For this review, take the finished solid that the model builds, in its own axes (mm). A direction names the side the tool comes from. Give positions to 0.01 mm unless a question says otherwise; leave off trailing zeros. Order: outer loops, then holes, each group sorted by start corner. A loop starts at its lowest first (then second) coordinate and runs counter-clockwise, first axis right, second up. Notation, with made-up numbers: M 57.5,-14 L 69.5,-14 A11 ccw 69.5,-8 Z; hole C -2,27.25 d3. An arc over 180 degrees is marked long. Use CSV: the item, a comma, the result in double quotes. Start each with the question number.
(1) Consider section B-B (x = 200). Give the number of separate pieces and of enclosed holes in the cut face, and give its area (3 significant figures).
(2) Consider section A-A (z = 32). Write out the cut boundary in (x, y), and give its area (3 significant figures).
(3) Consider section C-C (y = -329.5). Write out the cut boundary in (x, z).
(4) Draft analysis for pull direction X (two halves, no side actions). For faces 4 (the face through (212.945, -24.43, -7.395)), 5 (the face through (191, -366, 40)), 6 (the face through (0, -202, 12)), 7 (the face through (188.077, -21.245, 12.325)), state which applies: pulls with the +X half, pulls with the -X half, needs draft (parallel to the pull), parting line crosses it, or undercut.
(5) Wall thickness on L1, parallel to Y at x = 200, z = 5; L2, parallel to Y at x = 200, z = 28.5; L3, parallel to X at y = -25, z = 34.75: over which ranges is each line inside the solid? List them lowest first. Write a range as from..to.
(6) Clearance check with flat-ended pins moving along their axes: P1, Ø10, axis at x = 357.5, z = -2, coming from the -Y side; P2, Ø1, axis at x = 60, y = -195.5, coming from the +Z side; P3, Ø4, axis at x = 187.5, y = -43.5, coming from the -Z side. State where each tip first meets the part, or that it passes through.
(7) Tool access review of faces 1 (the face through (204.336, -394.524, 32.605)), 2 (the face through (219.98, -24.12, -7.39)), 3 (the face through (191, -366, -15)): name each direction out of +Z, -Z, +X, -X, +Y, -Y from which nothing blocks a thin tool from reaching the whole face with its end or side.
(8) Consider section D-D (x = 327). Write out the cut boundary in (y, z), and give its area (3 significant figures).
```python
from build123d import *

# Parameters (mm, degrees)
SKETCH1_W                = 400
SKETCH1_H                = 400
BOSS_EXTRUDE1_DEPTH      = 25
FILLET1_R                = 25
SKETCH2_R                = 12.5
CUT_EXTRUDE1_DEPTH       = 25
BOSS_EXTRUDE2_DEPTH      = 15
BOSS_EXTRUDE2_DEPTH_BACK = 40
SKETCH3_R                = 20
SKETCH3_R_2              = 12.957739805
SKETCH3_R_3              = 12.5


with BuildPart() as part:
    # Sketch1 → Boss-Extrude1 (new body)
    with BuildSketch(Plane.XY):
        with Locations((200, -200)):
            Rectangle(SKETCH1_W, SKETCH1_H)
    extrude(amount=BOSS_EXTRUDE1_DEPTH)

    # Fillet1
    fillet1_edges = [part.edges().sort_by_distance(p)[0] for p in [
        (0, 0, 12.5),
        (400, 0, 12.5),
        (400, -400, 12.5),
        (0, -400, 12.5),
    ]]
    fillet(fillet1_edges, radius=FILLET1_R)

    # Sketch2 → Cut-Extrude1 (cut)
    with BuildSketch(Plane(origin=(0, 0, 0), x_dir=(-1, 0, 0), z_dir=(0, 0, -1))):
        with Locations((-200, -25)):
            Circle(SKETCH2_R)
        with Locations((-200, -375)):
            Circle(SKETCH2_R)
    extrude(amount=-CUT_EXTRUDE1_DEPTH, mode=Mode.SUBTRACT)

    # Sketch3 → Boss-Extrude2 (add, two sides: drawn at the far end of the back side and taken through both)
    # profile 1 of 2: a face of its own
    with BuildSketch(Plane(origin=(0, 0, 0), x_dir=(-1, 0, 0), z_dir=(0, 0, -1)).offset(-BOSS_EXTRUDE2_DEPTH_BACK)):
        with Locations((-200, -25)):
            Circle(SKETCH3_R)
        with Locations((-200, -25)):
            Circle(SKETCH3_R_2, mode=Mode.SUBTRACT)
    # profile 2 of 2: a face of its own
    with BuildSketch(Plane(origin=(0, 0, 0), x_dir=(-1, 0, 0), z_dir=(0, 0, -1)).offset(-BOSS_EXTRUDE2_DEPTH_BACK)):
        with Locations((-200, -375)):
            Circle(SKETCH3_R)
        with Locations((-200, -375)):
            Circle(SKETCH3_R_3, mode=Mode.SUBTRACT)
    extrude(amount=BOSS_EXTRUDE2_DEPTH + BOSS_EXTRUDE2_DEPTH_BACK)


solid = part.part
```
Check result:
1,separate pieces,"3"
1,enclosed holes,"0"
1,area,"9,620 mm^2"
2,outline,"C 200,-375 d40; C 200,-25 d40; hole C 200,-25 d25.92; hole C 200,-375 d25"
2,area,"1,490 mm^2"
3,outline,"M 0,0 L 400,0 L 400,25 L 0,25 Z"
4,face 4,"undercut"
4,face 5,"needs draft"
4,face 6,"pulls with the -X half"
4,face 7,"undercut"
5,L1,"y = -400..-387.5, -362.5..-37.5, -12.5..0"
5,L2,"y = -395..-387.5, -362.5..-355, -45..-37.96, -12.04..-5"
5,L3,"x = 180..187.04, 212.96..220"
6,P1,"stops at y = -400"
6,P2,"stops at z = 25"
6,P3,"stops at z = 0"
7,face 1,"+Z"
7,face 2,"-Z"
7,face 3,"-Z, +X, -X, +Y, -Y"
8,outline,"M -400,0 L 0,0 L 0,25 L -400,25 Z"
8,area,"10,000 mm^2"
